```python
from build123d import *

# Parameters (mm, degrees)
EXTRUDE1_DEPTH = 60
SKETCH2_R      = 3
EXTRUDE2_DEPTH = 2
SKETCH3_R      = 1.5
EXTRUDE4_DEPTH = 61.336556083


with BuildPart() as part:
    # Sketch1 → Extrude1 (new body)
    with BuildSketch(Plane.XY):
        Polygon((4.5, 6.5), (-4.5, 6.5), (-4.5, 5.5), (-3.5, 5.5), (-3.5, 4.5), (-4.5, 4.5), (-4.5, 0), (4.5, 0), (4.5, 4.5), (3.5, 4.5), (3.5, 5.5), (4.5, 5.5), align=None)
    extrude(amount=EXTRUDE1_DEPTH)

    # Sketch2 → Extrude2 (cut)
    with BuildSketch(Plane(origin=(0, 6.5, 0), x_dir=(1, 0, 0), z_dir=(0, 1, 0))):
        with Locations(Location((0, -10, 0), (0, 0, 270))):
            Circle(SKETCH2_R)
        with Locations(Location((0, -30, 0), (0, 0, 270))):
            Circle(SKETCH2_R)
        with Locations(Location((0, -50, 0), (0, 0, 270))):
            Circle(SKETCH2_R)
        with Locations((0, -70)):
            Circle(SKETCH2_R)
        with Locations((0, -90)):
            Circle(SKETCH2_R)
        with Locations((0, -110)):
            Circle(SKETCH2_R)
        with Locations((0, -130)):
            Circle(SKETCH2_R)
        with Locations((0, -150)):
            Circle(SKETCH2_R)
        with Locations((0, -170)):
            Circle(SKETCH2_R)
        with Locations((0, -190)):
            Circle(SKETCH2_R)
        with Locations((0, -210)):
            Circle(SKETCH2_R)
        with Locations((0, -230)):
            Circle(SKETCH2_R)
        with Locations((0, -250)):
            Circle(SKETCH2_R)
        with Locations((0, -270)):
            Circle(SKETCH2_R)
        with Locations((0, -290)):
            Circle(SKETCH2_R)
        with Locations((0, -310)):
            Circle(SKETCH2_R)
        with Locations((0, -330)):
            Circle(SKETCH2_R)
        with Locations((0, -350)):
            Circle(SKETCH2_R)
        with Locations((0, -370)):
            Circle(SKETCH2_R)
        with Locations((0, -390)):
            Circle(SKETCH2_R)
        with Locations((0, -410)):
            Circle(SKETCH2_R)
        with Locations((0, -430)):
            Circle(SKETCH2_R)
        with Locations((0, -450)):
            Circle(SKETCH2_R)
        with Locations((0, -470)):
            Circle(SKETCH2_R)
        with Locations((0, -490)):
            Circle(SKETCH2_R)
        with Locations((0, -510)):
            Circle(SKETCH2_R)
        with Locations((0, -530)):
            Circle(SKETCH2_R)
        with Locations((0, -550)):
            Circle(SKETCH2_R)
        with Locations((0, -570)):
            Circle(SKETCH2_R)
        with Locations((0, -590)):
            Circle(SKETCH2_R)
        with Locations((0, -610)):
            Circle(SKETCH2_R)
        with Locations((0, -630)):
            Circle(SKETCH2_R)
    extrude(amount=-EXTRUDE2_DEPTH, mode=Mode.SUBTRACT)

    # Sketch3 → Extrude4 (cut, through all)
    with BuildSketch(Plane(origin=(0, 4.5, 0), x_dir=(1, 0, 0), z_dir=(0, 1, 0))):
        with Locations(Location((0, -10, 0), (0, 0, 270))):
            Circle(SKETCH3_R)
        with Locations(Location((0, -30, 0), (0, 0, 270))):
            Circle(SKETCH3_R)
        with Locations(Location((0, -50, 0), (0, 0, 270))):
            Circle(SKETCH3_R)
        with Locations((0, -70)):
            Circle(SKETCH3_R)
        with Locations((0, -90)):
            Circle(SKETCH3_R)
        with Locations((0, -110)):
            Circle(SKETCH3_R)
        with Locations((0, -130)):
            Circle(SKETCH3_R)
        with Locations((0, -150)):
            Circle(SKETCH3_R)
        with Locations((0, -170)):
            Circle(SKETCH3_R)
        with Locations((0, -190)):
            Circle(SKETCH3_R)
        with Locations((0, -210)):
            Circle(SKETCH3_R)
        with Locations((0, -230)):
            Circle(SKETCH3_R)
        with Locations((0, -250)):
            Circle(SKETCH3_R)
        with Locations((0, -270)):
            Circle(SKETCH3_R)
        with Locations((0, -290)):
            Circle(SKETCH3_R)
        with Locations((0, -310)):
            Circle(SKETCH3_R)
        with Locations((0, -330)):
            Circle(SKETCH3_R)
        with Locations((0, -350)):
            Circle(SKETCH3_R)
        with Locations((0, -370)):
            Circle(SKETCH3_R)
        with Locations((0, -390)):
            Circle(SKETCH3_R)
        with Locations((0, -410)):
            Circle(SKETCH3_R)
        with Locations((0, -430)):
            Circle(SKETCH3_R)
        with Locations((0, -450)):
            Circle(SKETCH3_R)
        with Locations((0, -470)):
            Circle(SKETCH3_R)
        with Locations((0, -490)):
            Circle(SKETCH3_R)
        with Locations((0, -510)):
            Circle(SKETCH3_R)
        with Locations((0, -530)):
            Circle(SKETCH3_R)
        with Locations((0, -550)):
            Circle(SKETCH3_R)
        with Locations((0, -570)):
            Circle(SKETCH3_R)
        with Locations((0, -590)):
            Circle(SKETCH3_R)
        with Locations((0, -610)):
            Circle(SKETCH3_R)
        with Locations((0, -630)):
            Circle(SKETCH3_R)
    extrude(amount=-EXTRUDE4_DEPTH, mode=Mode.SUBTRACT)


solid = part.part
```
Verification items for the finished model (mm, model axes). A direction names the side the tool comes from. Coordinates: 2 decimals unless noted, no trailing zeros. Write each loop counter-clockwise with the first axis right and the second up, starting at its lowest first coordinate (ties: lowest second). Pieces come first, ordered by that corner, then holes. Notation, with made-up numbers: M -34,41 L -9,41 A25 ccw -9,70 Z; hole C 27.25,8.25 d10. An arc over 180 degrees is marked long. One line per item, written item: value.
Item 1: Section check B-B, the plane y = 5. Record the boundary of the cut face in (x, z).
Check sheet entries:
outline: M -3.5,0 L 3.5,0 L 3.5,60 L -3.5,60 Z; hole C 0,10 d6; hole C 0,30 d6; hole C 0,50 d6
Item 2: Section check A-A, the plane x = 0. Record the boundary of the cut face in (y, z).
Check sheet entries:
outline: M 0,0 L 6.5,0 L 6.5,7 L 4.5,7 L 4.5,8.5 L 0,8.5 Z; M 0,11.5 L 4.5,11.5 L 4.5,13 L 6.5,13 L 6.5,27 L 4.5,27 L 4.5,28.5 L 0,28.5 Z; M 0,31.5 L 4.5,31.5 L 4.5,33 L 6.5,33 L 6.5,47 L 4.5,47 L 4.5,48.5 L 0,48.5 Z; M 0,51.5 L 4.5,51.5 L 4.5,53 L 6.5,53 L 6.5,60 L 0,60 Z
Item 3: Section check C-C, the plane z = 30. Record the boundary of the cut face in (x, y), plus the area to 3 significant figures.
Check sheet entries:
outline: M -4.5,0 L -1.5,0 L -1.5,4.5 L -3,4.5 L -3,6.5 L -4.5,6.5 L -4.5,5.5 L -3.5,5.5 L -3.5,4.5 L -4.5,4.5 Z; M 1.5,0 L 4.5,0 L 4.5,4.5 L 3.5,4.5 L 3.5,5.5 L 4.5,5.5 L 4.5,6.5 L 3,6.5 L 3,4.5 L 1.5,4.5 Z
area: 31.0 mm^2
Item 4: Mould release check, pull along X, two halves, no side actions. Record for faces 1 (the flat face through (-4.5, 2, 30)), 2 (the cylindrical face through (0.07, 2.28, 8.5)), 3 (the flat face through (4.5, 2, 30)): pulls with the +X half, pulls with the -X half, needs draft (parallel to the pull), parting line crosses it, or undercut.
Check sheet entries:
face 1: pulls with the -X half
face 2: undercut
face 3: pulls with the +X half
Item 5: Scan lines: line 1 along X through (y, z) = (5, 10); line 2 along X through (y, z) = (3.1, 30); line 3 along Z through (x, y) = (-0.25, 1). Record each from-to range of solid material in increasing order.
Check sheet entries:
line 1: x = -3.5 to -3, 3 to 3.5
line 2: x = -4.5 to -1.5, 1.5 to 4.5
line 3: z = 0 to 8.52, 11.48 to 28.52, 31.48 to 48.52, 51.48 to 60
Item 6: Access from +Z, -Z, +X, -X, +Y, -Y to the whole of each face (thin tool, end or side, straight path). Record for faces 4 (the flat face through (4, 5.5, 30)), 5 (the cylindrical face through (0, 6, 47)), 6 (the flat face through (0, 3, 0)), 7 (the flat face through (-4, 5.5, 30)).
Check sheet entries:
face 4: +Z, -Z, +X
face 5: +Y
face 6: -Z, +X, -X, +Y, -Y
face 7: +Z, -Z, -X
Item 7: Section check D-D, the plane z = 23.5. Record the boundary of the cut face in (x, y), plus the area to 3 significant figures.
Check sheet entries:
outline: M -4.5,0 L 4.5,0 L 4.5,4.5 L 3.5,4.5 L 3.5,5.5 L 4.5,5.5 L 4.5,6.5 L -4.5,6.5 L -4.5,5.5 L -3.5,5.5 L -3.5,4.5 L -4.5,4.5 Z
area: 56.5 mm^2
Item 8: Gauge pin test, flat ends, axial feed: pin 1 Ø0.8 at (y, z) = (5, 17.5) entering from -X; pin 2 Ø1.8 at (x, z) = (1.5, 50) entering from +Y. Record the tip position at first contact, or that the pin passes through.
Check sheet entries:
pin 1: stops at x = -3.5
pin 2: stops at y = 4.5
